Check sheet for the modelled part. Datum: model origin and axes. Units: mm. A direction names the side the tool comes from. Give positions to 0.01 mm unless a question says otherwise; leave off trailing zeros. Write each loop counter-clockwise with the first axis right and the second up, starting at its lowest first coordinate (ties: lowest second). Pieces come first, ordered by that corner, then holes.
from build123d import *

# Parameters (mm, degrees)
SALIENTE_EXTRUIR1_DEPTH = 1


with BuildPart() as part:
    # Croquis1 → Saliente-Extruir1 (new body)
    with BuildSketch(Plane.XY):
        with BuildLine():
            Line((-0.795495129, -7.079504871), (-1.856155301, -6.018844699))
            ThreePointArc((-1.856155301, -6.018844699), (2.425183773, -6.87045599), (0, -10.5))
            ThreePointArc((0, -10.5), (-9.700735091, -4.01817604), (-7.424621202, 7.424621202))
            Line((-7.424621202, 7.424621202), (-6.363961031, 6.363961031))
            ThreePointArc((-6.363961031, 6.363961031), (-8.314915793, -3.444150891), (0, -9))
            ThreePointArc((0, -9), (1.039364474, -7.444481139), (-0.795495129, -7.079504871))
        make_face()
    saliente_extruir1 = extrude(amount=SALIENTE_EXTRUIR1_DEPTH)

    # Simetría1: Saliente-Extruir1 across plane
    add(saliente_extruir1.mirror(Plane(origin=(-6.363961031, 6.363961031, 1), x_dir=(0, 0, 1), z_dir=(-0.7071067811865474, -0.7071067811865478, 0))))


solid = part.part
1) Access from +Z, -Z, +X, -X, +Y, -Y to the whole of each face (thin tool, end or side, straight path). Record for faces 1 (the flat face through (0, -5.5, 1)), 2 (the flat face through (-1.318, -6.557, 0.493)).
2) Scan lines: L1, parallel to Y at x = 1, z = 0.55; L2, parallel to Y at x = 0.25, z = 0.6; L3, parallel to X at y = -7, z = 0.7 (3 decimals). Record each from-to range of solid material in increasing order.
3) Draft check along X on faces 3 (the flat face through (6.557, 1.318, 0.493)), 4 (the flat face through (0, -5.5, 0)). Enter one of: +X half, -X half, draft (parallel to the pull), parting line (faces both ways), or undercut.
4) Sectioned sample at A-A on x = 5.75. Record the boundary of the cut face in (y, z).
5) Sectioned sample at D-D on x = -0.5. Record the boundary of the cut face in (y, z).
6) Sectioned sample at C-C on y = 3.75. Record the boundary of the cut face in (x, z), then the cut area to 3 significant figures.
Answers below:
1. face 1: +Z, +X, -X, +Y, -Y
1. face 2: +Z, -Z
2. L1: y = -10.3 to -8.39, -7.36 to -5.45, 8.94 to 10.45
2. L2: y = -10.49 to -8.97, -6.78 to -5.26, 9 to 10.5
2. L3: x = -7.826 to -5.657, -0.875 to -0.707, 0.707 to 2.475
3. face 3: undercut
3. face 4: draft
4. outline: (-1.54, 0) - (1.54, 0) - (1.54, 1) - (-1.54, 1) - close; (6.92, 0) - (8.79, 0) - (8.79, 1) - (6.92, 1) - close
5. outline: (-10.49, 0) - (-8.99, 0) - (-8.99, 1) - (-10.49, 1) - close; (-6.87, 0) - (-5.3, 0) - (-5.3, 1) - (-6.87, 1) - close; (8.99, 0) - (10.49, 0) - (10.49, 1) - (8.99, 1) - close
6. outline: (-9.81, 0) - (-8.18, 0) - (-8.18, 1) - (-9.81, 1) - close; (8.18, 0) - (9.81, 0) - (9.81, 1) - (8.18, 1) - close
6. area: 3.25 mm2
